Source: CAD feature listing. Evaluate the final solid. Frame: model axes, mm. Give positions to 0.01 mm unless a question says otherwise; leave off trailing zeros. Order: outer loops, then holes, each group sorted by start corner. A loop starts at its lowest first (then second) coordinate and runs counter-clockwise, first axis right, second up.
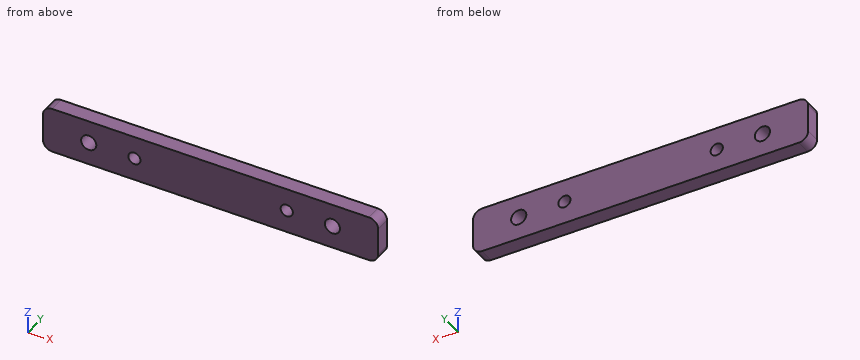
from build123d import *

# Parameters (mm, degrees)
SKETCH_1_W          = 110
SKETCH_1_H          = 15
EXTRUDE_1_DEPTH     = 5
FILLET_1_R          = 3
SKETCH_2_R          = 2.5
SKETCH_2_R_2        = 2
CUT_EXTRUDE_1_DEPTH = 5


with BuildPart() as part:
    # 草图1 → 凸台-拉伸1 (new body)
    with BuildSketch(Plane(origin=(0, 0, 0), x_dir=(1, 0, 0), z_dir=(0, 1, 0))):
        Rectangle(SKETCH_1_W, SKETCH_1_H)
    extrude(amount=EXTRUDE_1_DEPTH)

    # 圆角1
    fillet_1_edges = [part.edges().sort_by_distance(p)[0] for p in [
        (55, 2.5, 7.5),
        (-55, 2.5, 7.5),
        (-55, 2.5, -7.5),
        (55, 2.5, -7.5),
    ]]
    fillet(fillet_1_edges, radius=FILLET_1_R)

    # 草图2 → 切除-拉伸1 (cut)
    with BuildSketch(Plane(origin=(0, 5, 0), x_dir=(1, 0, 0), z_dir=(0, 1, 0))):
        with Locations(Location((40, 0, 0), (0, 0, 270))):
            Circle(SKETCH_2_R)
        with Locations(Location((25, 0, 0), (0, 0, 270))):
            Circle(SKETCH_2_R_2)
        with Locations(Location((-40, 0, 0), (0, 0, 90))):
            Circle(SKETCH_2_R)
        with Locations(Location((-25, 0, 0), (0, 0, 90))):
            Circle(SKETCH_2_R_2)
    extrude(amount=-CUT_EXTRUDE_1_DEPTH, mode=Mode.SUBTRACT)


solid = part.part
1) Section query B-B on x = 40. Output: boundary loops of the cut face in (y, z).
Checks:
outline: (0, -7.5) - (5, -7.5) - (5, -2.5) - (0, -2.5) - close; (0, 2.5) - (5, 2.5) - (5, 7.5) - (0, 7.5) - close
2) Section query C-C on z = -1. Output: boundary loops of the cut face in (x, y).
Checks:
outline: (-55, 0) - (-42.29, 0) - (-42.29, 5) - (-55, 5) - close; (-37.71, 0) - (-26.73, 0) - (-26.73, 5) - (-37.71, 5) - close; (-23.27, 0) - (23.27, 0) - (23.27, 5) - (-23.27, 5) - close; (26.73, 0) - (37.71, 0) - (37.71, 5) - (26.73, 5) - close; (42.29, 0) - (55, 0) - (55, 5) - (42.29, 5) - close
3) Ray query, L1, parallel to X at y = 4.85, z = -0.25; L2, parallel to Z at x = 40.5, y = 1.95; L3, parallel to Z at x = -24, y = 0.35. Return the intervals inside material, ascending.
Checks:
L1: x = -55 to -42.49, -37.51 to -26.98, -23.02 to 23.02, 26.98 to 37.51, 42.49 to 55
L2: z = -7.5 to -2.45, 2.45 to 7.5
L3: z = -7.5 to -1.73, 1.73 to 7.5
4) Section query A-A on y = 3.7. Output: boundary loops of the cut face in (x, z).
Checks:
outline: (-55, -4.5) arc R3 ccw to (-52, -7.5) - (52, -7.5) arc R3 ccw to (55, -4.5) - (55, 4.5) arc R3 ccw to (52, 7.5) - (-52, 7.5) arc R3 ccw to (-55, 4.5) - close; hole circle Ø5 at (-40, 0); hole circle Ø4 at (-25, 0); hole circle Ø4 at (25, 0); hole circle Ø5 at (40, 0)
5) First-contact query: pin 1 Ø3.5 at (x, z) = (-25, 0) entering from +Y; pin 2 Ø1.5 at (y, z) = (4, 5.5) entering from -X. Flat tips, straight axial feed; report the tip coordinate or a pass-through.
Checks:
pin 1: passes through
pin 2: stops at x = -54.99
6) Section query D-D on x = 25. Output: boundary loops of the cut face in (y, z).
Checks:
outline: (0, -7.5) - (5, -7.5) - (5, -2) - (0, -2) - close; (0, 2) - (5, 2) - (5, 7.5) - (0, 7.5) - close
